Part model, mm, in its own coordinate system. Give positions to 0.01 mm unless a question says otherwise; leave off trailing zeros. Write each loop counter-clockwise with the first axis right and the second up, starting at its lowest first coordinate (ties: lowest second). Pieces come first, ordered by that corner, then holes. Notation, with made-up numbers: (21, 89.25) - (76, 89.25) arc R19 ccw to (76, 120.25) - close; hole circle Ø8 at (3, 52.5). An arc over 180 degrees is marked (long way). Answer as a JSON object with one key per item and string values. Group by question number.
```python
from build123d import *

# Parameters (mm, degrees)
SKETCH2_W          = 70
SKETCH2_H          = 44
EXTRUDE1_DEPTH     = 600
CUT_EXTRUDE1_REACH = 607.67
SKETCH3_R          = 5


with BuildPart() as part:
    # Sketch2 → Extrude1 (new body)
    with BuildSketch(Plane.XY):
        with Locations((35, 22)):
            Rectangle(SKETCH2_W, SKETCH2_H)
    extrude(amount=EXTRUDE1_DEPTH)

    # Sketch3 → Cut-Extrude1 (cut, up to next)
    with BuildSketch(Plane(origin=(0, 44, 0), x_dir=(-1, 0, 0), z_dir=(0, 1, 0)), mode=Mode.PRIVATE) as cut_extrude1_sk1:
        with Locations(Location((-34.89201671, 200, 0), (0, 0, 90))):
            Circle(SKETCH3_R)
    cut_extrude1_tool1 = extrude(cut_extrude1_sk1.sketch, amount=-CUT_EXTRUDE1_REACH, mode=Mode.PRIVATE) & part.part
    add(cut_extrude1_tool1.solids().sort_by_distance((34.892017, 44, 200))[0], mode=Mode.SUBTRACT)


solid = part.part
```
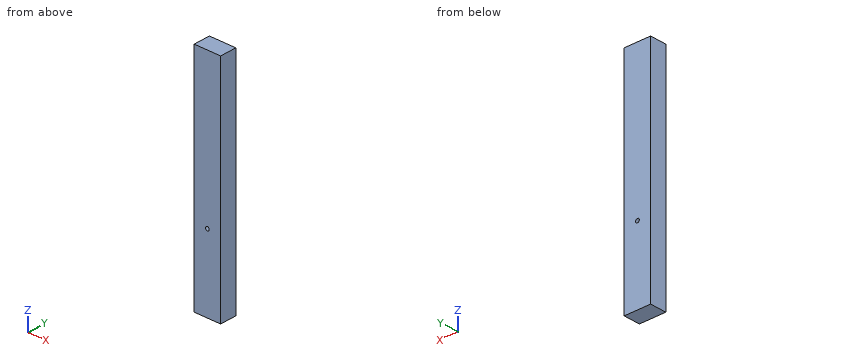
1) Probe line 1 (X direction, y = 24, z = 200); line 2 (Z direction, x = 33, y = 25); line 3 (Z direction, x = 36.5, y = 21). List the from-to ranges inside material, lowest first.
2) Drop a flat-ended pin along its axis: P1, Ø3, axis at x = 62.5, y = 17, coming from the -Z side. Give the stop position or say it passes through.
3) Band-saw the part on A-A (z = 200). List the corners of the cut face in (x, y), plus the area to 3 significant figures.
Verdict:
{
 "1": {"line 1": "0 to 29.89, 39.89 to 70", "line 2": "0 to 195.37, 204.63 to 600", "line 3": "0 to 195.27, 204.73 to 600"},
 "2": {"P1": "z = 0"},
 "3": {"outline": "(0, 0) - (29.89, 0) - (29.89, 44) - (0, 44) - close; (39.89, 0) - (70, 0) - (70, 44) - (39.89, 44) - close", "area": "2,640 mm2"}
}
